Geometry check sheet. Reference: the model listing, model coordinates, mm. Face numbers are marked on the shaded views. A direction names the side the tool comes from. Give positions to 0.01 mm unless a question says otherwise; leave off trailing zeros. Loops run counter-clockwise (first coordinate to the right, second up) from the corner with the lowest first, then second, coordinate; pieces in that order, holes last.
1. Material ranges on L1, parallel to X at y = 3.5, z = 0; L2, parallel to X at y = 3.5, z = -23; L3, parallel to Z at x = -26.5, y = 5.25, recorded low to high.
2. Release check for a two-part mould opening along X. For the marked faces 1, 2, 3 and 4 record: +X half, -X half, draft (parallel to the pull), parting line (faces both ways), or undercut.
3. Cross-section at C-C, the plane x = 31.5. Record the cut outline in (y, z).
4. Go/stop test with flat-tipped pins: pin 1 Ø3 at (x, z) = (-0.5, -13.5) entering from -Y; pin 2 Ø1.9 at (y, z) = (2, 22.5) entering from +X; pin 3 Ø3 at (y, z) = (4.5, -21) entering from -X; pin 4 Ø1.9 at (x, y) = (7, 2) entering from -Z. Record where each tip stops, or that it passes through.
5. Cross-section at B-B, the plane y = 1.75. State how many separate pieces and enclosed holes the cut face has, plus the area to 3 significant figures.
6. Tool access check on the marked faces 5, 6, 7 and 8. Record the directions out of +Z, -Z, +X, -X, +Y, -Y that give a thin tool (end or side, any length) a straight path to the whole face; none if there is none.
7. Cross-section at A-A, the plane z = 0. Record the cut outline in (x, y), plus the area to 3 significant figures.
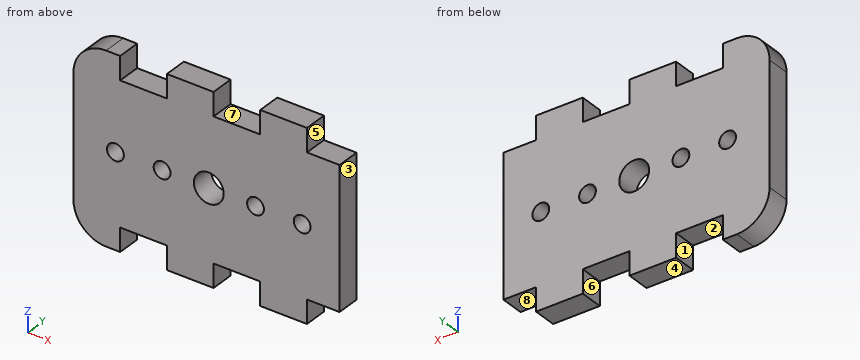
from build123d import *

# Parameters (mm, degrees)
MAIN_DEPTH             = 6.35
SKETCH3_R              = 4.064
SKETCH3_R_2            = 2.286
GEAR_MOUNT_HOLES_DEPTH = 51.497474194
SKETCH4_W              = 5.978415147
SKETCH4_H              = 38.1
SKETCH4_W_2            = 8.0137
CUT_EXTRUDE2_DEPTH     = 51.497474194
FILLET1_R              = 8.89


with BuildPart() as part:
    # Sketch1 → Main (new body)
    with BuildSketch(Plane(origin=(0, 0, 0), x_dir=(1, 0, 0), z_dir=(0, 1, 0))):
        Polygon((-43.18, 19.05), (-35.1663, 19.05), (-35.1663, 25.4), (-22.4663, 25.4), (-22.4663, 19.05), (-9.7663, 19.05), (-9.7663, 25.4), (2.9337, 25.4), (2.9337, 19.05), (15.6337, 19.05), (15.6337, 25.4), (28.3337, 25.4), (28.3337, 19.05), (43.18, 19.05), (43.18, -19.05), (28.3337, -19.05), (28.3337, -25.4), (15.6337, -25.4), (15.6337, -19.05), (2.9337, -19.05), (2.9337, -25.4), (-9.7663, -25.4), (-9.7663, -19.05), (-22.4663, -19.05), (-22.4663, -25.4), (-35.1663, -25.4), (-35.1663, -19.05), (-43.18, -19.05), align=None)
    extrude(amount=MAIN_DEPTH)

    # Sketch3 → Gear Mount Holes (cut, through all)
    with BuildSketch(Plane(origin=(0, 6.35, 0), x_dir=(1, 0, 0), z_dir=(0, 1, 0))):
        with Locations(Location((1.641584853, 0, 0), (0, 0, 270))):
            Circle(SKETCH3_R)
        with Locations(Location((14.341584853, 0, 0), (0, 0, 270))):
            Circle(SKETCH3_R_2)
        with Locations(Location((27.041584853, 0, 0), (0, 0, 270))):
            Circle(SKETCH3_R_2)
        with Locations(Location((-11.058415147, 0, 0), (0, 0, 270))):
            Circle(SKETCH3_R_2)
        with Locations(Location((-23.758415147, 0, 0), (0, 0, 270))):
            Circle(SKETCH3_R_2)
    extrude(amount=-GEAR_MOUNT_HOLES_DEPTH, mode=Mode.SUBTRACT)

    # Sketch4 → Cut-Extrude2 (cut, through all)
    with BuildSketch(Plane(origin=(0, 6.35, 0), x_dir=(1, 0, 0), z_dir=(0, 1, 0))):
        with Locations((40.190792426, 0)):
            Rectangle(SKETCH4_W, SKETCH4_H)
        with Locations((-39.17315, 0)):
            Rectangle(SKETCH4_W_2, SKETCH4_H)
    extrude(amount=-CUT_EXTRUDE2_DEPTH, mode=Mode.SUBTRACT)

    # Fillet1
    fillet1_edges = [part.edges().sort_by_distance(p)[0] for p in [
        (-35.1663, 3.175, -25.4),
        (-35.1663, 3.175, 25.4),
    ]]
    fillet(fillet1_edges, radius=FILLET1_R)


solid = part.part
Result:
1. L1: x = -35.17 to -26.04, -21.47 to -13.34, -8.77 to -2.42, 5.71 to 12.06, 16.63 to 24.76, 29.33 to 37.2
1. L2: x = -32.35 to -22.47, -9.77 to 2.93, 15.63 to 28.33
1. L3: z = -25.4 to 25.4
2. face 1: undercut
2. face 2: undercut
2. face 3: +X half
2. face 4: draft
3. outline: (0, -19.05) - (6.35, -19.05) - (6.35, 19.05) - (0, 19.05) - close
4. pin 1: stops at y = 0
4. pin 2: stops at x = 28.33
4. pin 3: stops at x = -34.65
4. pin 4: stops at z = -19.05
5. separate pieces: 1
5. enclosed holes: 5
5. area: 3,090 mm2
6. face 5: +Z, +X, +Y, -Y
6. face 6: -Z, +Y, -Y
6. face 7: +Z, +Y, -Y
6. face 8: -Z, +X, +Y, -Y
7. outline: (-35.17, 0) - (-26.04, 0) - (-26.04, 6.35) - (-35.17, 6.35) - close; (-21.47, 0) - (-13.34, 0) - (-13.34, 6.35) - (-21.47, 6.35) - close; (-8.77, 0) - (-2.42, 0) - (-2.42, 6.35) - (-8.77, 6.35) - close; (5.71, 0) - (12.06, 0) - (12.06, 6.35) - (5.71, 6.35) - close; (16.63, 0) - (24.76, 0) - (24.76, 6.35) - (16.63, 6.35) - close; (29.33, 0) - (37.2, 0) - (37.2, 6.35) - (29.33, 6.35) - close
7. area: 292 mm2
